For this review, take the finished solid that the model builds, in its own axes (mm). Give positions to 0.01 mm unless a question says otherwise; leave off trailing zeros. Write each loop counter-clockwise with the first axis right and the second up, starting at its lowest first coordinate (ties: lowest second). Pieces come first, ordered by that corner, then holes.
1) We need section B-B on x = 88.9. Give the boundary of the cut face in (y, z) (3 decimals).
2) Draft analysis for pull direction X (two halves, no side actions). For faces 1 (the face through (88, 90, 0)), 2 (the face through (26.85, 39.99, 1.57)), state which applies: pulls with the +X half, pulls with the -X half, needs draft (parallel to the pull), parting line crosses it, or undercut.
3) We need section A-A on x = 152.4. Give the number of separate pieces and of enclosed holes in the cut face, and give its area (3 significant figures).
4) We need section C-C on y = 165.1. Give the boundary of the cut face in (x, z) (3 decimals), and give its area (3 significant figures).
5) For P1, Ø6, axis at x = 108, y = 89, coming from the -Z side, flat-tipped, find the tip position at first contact; note if it passes through.
6) Wall thickness on line 1 along X through (y, z) = (139.7, 1.95); line 2 along X through (y, z) = (14, 2.7); line 3 along X through (y, z) = (114.3, 2.35): over which ranges is each line inside the solid? List them lowest first.
Autodesk Inventor part; units mm, degrees
ref_plane "YZ Plane" through (0, 0, 0) normal (1, 0, 0) x (0, 1, 0)
ref_plane "XZ Plane" through (0, 0, 0) normal (0, 1, 0) x (-1, 0, 0)
ref_plane "XY Plane" through (0, 0, 0) normal (0, 0, 1) x (1, 0, 0)
sketch "Sketch1" plane through (0, 0, 0) normal (0, 0, 1) x (1, 0, 0)
  line L0 (0, 0) -> (177.8, 0)
  line L1 (177.8, 0) -> (177.8, 177.8)
  line L2 (177.8, 177.8) -> (0, 177.8)
  line L3 (0, 177.8) -> (0, 0)
  dimension "d0" = 177.8
  dimension "d1" = 177.8
extrude "Extrusion1" add sketch "Sketch1" along normal blind 3.175
sketch "Sketch2" plane through (0, 0, 3.175) normal (0, 0, 1) x (1, 0, 0)
  line L0 (0, 0) -> (177.8, 0)
  line L1 (177.8, 0) -> (177.8, 177.8)
  line L2 (177.8, 177.8) -> (0, 177.8) construction
  line L3 (0, 177.8) -> (0, 0)
  line L4 (177.8, 177.8) -> (0, 177.8) construction
  line L5 (88.9, 177.8) -> (76.2, 177.8) construction
  line L6 (88.9, 177.8) -> (101.6, 177.8) construction
  line L7 (76.2, 177.8) -> (76.2, 127) construction
  line L8 (76.2, 127) -> (101.6, 127) construction
  line L9 (101.6, 177.8) -> (101.6, 127) construction
  line L10 (88.9, 127) -> (88.9, 107.95) construction
  circle A0 centre (88.9, 117.475) radius 9.525 construction
  circle A1 centre (88.9, 117.475) radius 7.874
  dimension "d4" = 12.7
  dimension "d5" = 12.7
  dimension "d6" = 50.8
  dimension "d7" = 19.05
  dimension "d8" = 15.748
extrude "Extrusion2" cut sketch "Sketch2" against normal through all
sketch "Sketch3" plane through (0, 0, 3.175) normal (0, 0, 1) x (1, 0, 0)
  circle A0 centre (88.9, 117.475) radius 7.874
  line L0 (0, 0) -> (177.8, 0)
  line L1 (177.8, 0) -> (177.8, 177.8)
  line L2 (177.8, 177.8) -> (0, 177.8)
  line L3 (0, 177.8) -> (0, 0)
  circle A1 centre (88.9, 117.475) radius 10.16 construction
  line L4 (88.9, 117.475) -> (88.9, 107.315) construction
  line L5 (88.9, 107.315) -> (88.9, 102.235) construction
  circle A2 centre (88.9, 102.235) radius 3.9116
  dimension "d11" = 20.32
  dimension "d12" = 5.08
  dimension "d13" = 7.8232
extrude "Extrusion3" cut sketch "Sketch3" against normal through all contours A2
sketch "Sketch4" plane through (0, 0, 3.175) normal (0, 0, 1) x (1, 0, 0)
  circle A0 centre (88.9, 102.235) radius 3.9116
  circle A1 centre (88.9, 117.475) radius 7.874
  line L0 (0, 0) -> (177.8, 0)
  line L1 (177.8, 0) -> (177.8, 177.8)
  line L2 (177.8, 177.8) -> (0, 177.8) construction
  line L3 (0, 177.8) -> (0, 0)
  line L4 (0, 177.8) -> (25.4, 177.8) construction
  line L5 (177.8, 177.8) -> (0, 177.8) construction
  line L6 (177.8, 177.8) -> (152.4, 177.8) construction
  line L7 (25.4, 177.8) -> (25.4, 152.4) construction
  line L8 (152.4, 177.8) -> (152.4, 152.4) construction
  circle A2 centre (25.4, 152.4) radius 2.3812
  circle A3 centre (152.4, 152.4) radius 2.3813
  line L9 (0, 165.1) -> (25.4, 165.1) construction
  line L10 (177.8, 165.1) -> (152.4, 165.1) construction
  line L11 (25.4, 165.1) -> (25.4, 139.7) construction
  line L12 (152.4, 165.1) -> (152.4, 139.7) construction
  circle A4 centre (25.4, 139.7) radius 2.3812
  line L13 (0, 152.4) -> (25.4, 152.4) construction
  line L14 (177.8, 152.4) -> (152.4, 152.4) construction
  line L15 (25.4, 152.4) -> (25.4, 127) construction
  line L16 (152.4, 152.4) -> (152.4, 127) construction
  circle A5 centre (25.4, 127) radius 2.3812
  line L17 (0, 139.7) -> (25.4, 139.7) construction
  line L18 (177.8, 139.7) -> (152.4, 139.7) construction
  line L19 (25.4, 139.7) -> (25.4, 114.3) construction
  line L20 (152.4, 139.7) -> (152.4, 114.3) construction
  circle A6 centre (25.4, 114.3) radius 2.3812
  line L21 (0, 127) -> (25.4, 127) construction
  line L22 (177.8, 127) -> (152.4, 127) construction
  line L23 (25.4, 127) -> (25.4, 101.6) construction
  line L24 (152.4, 127) -> (152.4, 101.6) construction
  circle A7 centre (25.4, 101.6) radius 2.3812
  line L25 (0, 114.3) -> (25.4, 114.3) construction
  line L26 (177.8, 114.3) -> (152.4, 114.3) construction
  line L27 (25.4, 114.3) -> (25.4, 88.9) construction
  line L28 (152.4, 114.3) -> (152.4, 88.9) construction
  circle A8 centre (25.4, 88.9) radius 2.3812
  line L29 (0, 101.6) -> (25.4, 101.6) construction
  line L30 (177.8, 101.6) -> (152.4, 101.6) construction
  line L31 (25.4, 101.6) -> (25.4, 76.2) construction
  line L32 (152.4, 101.6) -> (152.4, 76.2) construction
  circle A9 centre (25.4, 76.2) radius 2.3812
  line L33 (0, 88.9) -> (25.4, 88.9) construction
  line L34 (177.8, 88.9) -> (152.4, 88.9) construction
  line L35 (25.4, 88.9) -> (25.4, 63.5) construction
  line L36 (152.4, 88.9) -> (152.4, 63.5) construction
  circle A10 centre (25.4, 63.5) radius 2.3812
  line L37 (0, 76.2) -> (25.4, 76.2) construction
  line L38 (177.8, 76.2) -> (152.4, 76.2) construction
  line L39 (25.4, 76.2) -> (25.4, 50.8) construction
  line L40 (152.4, 76.2) -> (152.4, 50.8) construction
  circle A11 centre (25.4, 50.8) radius 2.3812
  line L41 (0, 63.5) -> (25.4, 63.5) construction
  line L42 (177.8, 63.5) -> (152.4, 63.5) construction
  line L43 (25.4, 63.5) -> (25.4, 38.1) construction
  line L44 (152.4, 63.5) -> (152.4, 38.1) construction
  circle A12 centre (25.4, 38.1) radius 2.3812
  line L45 (0, 50.8) -> (25.4, 50.8) construction
  line L46 (177.8, 50.8) -> (152.4, 50.8) construction
  line L47 (25.4, 50.8) -> (25.4, 25.4) construction
  line L48 (152.4, 50.8) -> (152.4, 25.4) construction
  circle A13 centre (25.4, 25.4) radius 2.3812
  line L49 (0, 38.1) -> (25.4, 38.1) construction
  line L50 (177.8, 38.1) -> (152.4, 38.1) construction
  line L51 (25.4, 38.1) -> (25.4, 12.7) construction
  line L52 (152.4, 38.1) -> (152.4, 12.7) construction
  circle A14 centre (25.4, 12.7) radius 2.3812
  circle A15 centre (152.4, 139.7) radius 2.3813
  circle A16 centre (152.4, 127) radius 2.3813
  circle A17 centre (152.4, 114.3) radius 2.3813
  circle A18 centre (152.4, 101.6) radius 2.3813
  circle A19 centre (152.4, 88.9) radius 2.3813
  circle A20 centre (152.4, 76.2) radius 2.3813
  circle A21 centre (152.4, 63.5) radius 2.3813
  circle A22 centre (152.4, 50.8) radius 2.3813
  circle A23 centre (152.4, 38.1) radius 2.3813
  circle A24 centre (152.4, 25.4) radius 2.3813
  circle A25 centre (152.4, 12.7) radius 2.3813
  circle A26 centre (25.4, 165.1) radius 2.3813
  circle A27 centre (152.4, 165.1) radius 2.3812
  dimension "d16" = 25.4
  dimension "d17" = 25.4
  dimension "d18" = 25.4
  dimension "d19" = 25.4
  dimension "d20" = 4.7625
  dimension "d21" = 4.7625
  dimension "d24" = 12.7
  dimension "d31" = 12.7
  dimension "d47" = 4.7625
  dimension "d48" = 4.7625
sketch "Sketch5" plane through (0, 0, 3.175) normal (0, 0, 1) x (1, 0, 0)
  circle A0 centre (88.9, 102.235) radius 3.9116 construction
  circle A1 centre (88.9, 117.475) radius 7.874 construction
  line L0 (0, 0) -> (177.8, 0) construction
  line L1 (177.8, 0) -> (177.8, 177.8) construction
  line L2 (177.8, 177.8) -> (0, 177.8) construction
  line L3 (0, 177.8) -> (0, 0) construction
  line L4 (177.8, 177.8) -> (0, 177.8) construction
  line L5 (88.9, 177.8) -> (76.2, 177.8) construction
  line L6 (88.9, 177.8) -> (101.6, 177.8) construction
  line L7 (76.2, 177.8) -> (25.4, 177.8)
  line L8 (101.6, 177.8) -> (152.4, 177.8)
  dimension "d43" = 12.7
  dimension "d44" = 12.7
  dimension "d45" = 50.8
  dimension "d46" = 50.8
hole "Hole2" at (25.4, 165.1, 3.175) at (152.4, 165.1, 3.175) at (25.4, 139.7, 3.175) at (25.4, 114.3, 3.175) at (25.4, 88.9, 3.175) at (25.4, 63.5, 3.175) at (25.4, 38.1, 3.175) at (25.4, 12.7, 3.175) at (152.4, 139.7, 3.175) at (152.4, 114.3, 3.175) at (152.4, 88.9, 3.175) at (152.4, 63.5, 3.175) at (152.4, 38.1, 3.175) at (152.4, 12.7, 3.175) direction (0, 0, -1) diameter 4.7625 end through all
properties part number "ClawPlate"
Results list:
1. outline: (0, 0) - (98.323, 0) - (98.323, 3.175) - (0, 3.175) - close; (106.147, 0) - (109.601, 0) - (109.601, 3.175) - (106.147, 3.175) - close; (125.349, 0) - (177.8, 0) - (177.8, 3.175) - (125.349, 3.175) - close
2. face 1: needs draft
2. face 2: undercut
3. separate pieces: 8
3. enclosed holes: 0
3. area: 459 mm2
4. outline: (0, 0) - (23.019, 0) - (23.019, 3.175) - (0, 3.175) - close; (27.781, 0) - (150.019, 0) - (150.019, 3.175) - (27.781, 3.175) - close; (154.781, 0) - (177.8, 0) - (177.8, 3.175) - (154.781, 3.175) - close
4. area: 534 mm2
5. P1: stops at z = 0
6. line 1: x = 0 to 23.02, 27.78 to 150.02, 154.78 to 177.8
6. line 2: x = 0 to 23.4, 27.4 to 150.4, 154.4 to 177.8
6. line 3: x = 0 to 23.02, 27.78 to 81.69, 96.11 to 150.02, 154.78 to 177.8
